Design review of the part built by this model. Coordinates are the model's own, in mm. A direction names the side the tool comes from. Coordinates: 2 decimals unless noted, no trailing zeros. Write each loop counter-clockwise with the first axis right and the second up, starting at its lowest first coordinate (ties: lowest second). Pieces come first, ordered by that corner, then holes. Notation, with made-up numbers: (-17, 84.25) -> (33, 84.25) arc R15 ccw to (33, 104.25) -> close; hole circle Ø4 at (76.25, 47.5). An arc over 180 degrees is marked (long way). Return JSON: item names as keys, results as strings. Group by question number.
from build123d import *

# Parameters (mm, degrees)
F0_R     = 3
F0_R_2   = 4.5
F1_DEPTH = 25


with BuildPart() as f1:
    # F0 (on Front) → F1 (new body)
    with BuildSketch(Plane.XZ):
        with BuildLine():
            ThreePointArc((10.9026810919, 60.0256923786), (-22.2558754476, 56.4666978044), (-51.1818335692, 39.870154161))
            ThreePointArc((-51.1818335692, 39.870154161), (-67.2310606154, 11.5408714989), (-71.6096891644, -20.7229403799))
            ThreePointArc((-71.6096891644, -20.7229403799), (-68.3273517642, -26.7421593589), (-61.4792606521, -27.0713766838))
            ThreePointArc((-61.4792606521, -27.0713766838), (-23.2487235956, -19.9089821225), (14.7948054645, -28.00612706))
            ThreePointArc((14.7948054645, -28.00612706), (34.09763812, -38.0650715452), (52.3656483576, -49.8998302939))
            ThreePointArc((52.3656483576, -49.8998302939), (55.6232730928, -50.3420263302), (57.6954634801, -47.7898344783))
            ThreePointArc((57.6954634801, -47.7898344783), (67.4841016349, -13.4719946795), (63.4264131289, 21.9831421749))
            ThreePointArc((63.4264131289, 21.9831421749), (41.7291215347, 47.3065311635), (10.9026810919, 60.0256923786))
        make_face()
        with Locations((-64.4427245231, -20.592329134)):
            Circle(F0_R, mode=Mode.SUBTRACT)
        with Locations((18.0438014374, -21.0330026143)):
            Circle(F0_R, mode=Mode.SUBTRACT)
        with Locations((-45.0222906279, 34.0597224955)):
            Circle(F0_R_2, mode=Mode.SUBTRACT)
        with BuildLine():
            add(Edge.make_bspline(
                [(-65.9818429495, -13.7766383887), (-64.3561406503, -13.9889919324), (-61.002475647, -14.4129805983), (-58.786662695, -17.3941098492), (-57.6425891256, -18.9315586575)],
                knots=[0, 0, 0, 0, 0.4837523045, 1, 1, 1, 1], degree=3))
            ThreePointArc((-65.9818429495, -13.7766383887), (-63.1199927656, 5.6889897511), (-55.6653674819, 23.8969393125))
            add(Edge.make_bspline(
                [(-55.6653674819, 23.8969393125), (-54.1157834703, 24.558722907), (-50.9743628562, 25.897077509), (-44.9169668051, 25.5411930836), (-44.499564984, 25.5987820264), (-44.4126954758, 25.6059592173)],
                knots=[0, 0, 0, 0, 0.4368464907, 0.8829086428, 1, 1, 1, 1], degree=3))
            ThreePointArc((-44.4126954758, 25.6059592173), (-38.3027773263, 28.8742935487), (-36.6900921562, 35.6131625664))
            add(Edge.make_bspline(
                [(-34.08346527, 45.6139450583), (-35.2318735073, 44.1052978146), (-37.495431158, 41.0832942182), (-36.9568434928, 37.4300314786), (-36.6900921562, 35.6131625664)],
                knots=[0, 0, 0, 0, 0.5034654691, 1, 1, 1, 1], degree=3))
            ThreePointArc((-34.08346527, 45.6139450583), (-21.4497726915, 51.0485334301), (-8.0636271487, 54.2038537692))
            add(Edge.make_bspline(
                [(-8.0636271487, 54.2038537692), (-5.1314488098, 53.9873966847), (0.3914162184, 53.5818086349), (3.3084081042, 49.9752607352), (4.6788664975, 48.2869338255)],
                knots=[0, 0, 0, 0, 0.5311112281, 1, 1, 1, 1], degree=3))
            ThreePointArc((4.6788664975, 48.2869338255), (8.9267083452, 46.2578656633), (13.5002491076, 47.3732144268))
            add(Edge.make_bspline(
                [(27.5275195375, 49.6756181297), (24.3589504651, 50.2644097694), (18.5753078163, 51.2779486411), (15.0780756623, 48.5877160028), (13.5002491076, 47.3732144268)],
                knots=[0, 0, 0, 0, 0.5497885765, 1, 1, 1, 1], degree=3))
            ThreePointArc((27.5275195375, 49.6756181297), (40.3031395338, 42.4916724249), (50.800144894, 32.2623801401))
            add(Edge.make_bspline(
                [(50.800144894, 32.2623801401), (51.3048604695, 30.5691603197), (52.2209505288, 27.262036777), (51.106083954, 24.3879103118), (50.5611791748, 22.9987592368)],
                knots=[0, 0, 0, 0, 0.5176067222, 1, 1, 1, 1], degree=3))
            ThreePointArc((50.5611791748, 22.9987592368), (50.2536306678, 17.192161847), (54.4628675293, 13.1804933194))
            add(Edge.make_bspline(
                [(61.7354629672, 6.576572241), (60.8612124825, 8.1098386582), (59.0540175823, 11.1146660647), (55.9863654121, 12.4994575374), (54.4628675293, 13.1804933194)],
                knots=[0, 0, 0, 0, 0.5060903587, 1, 1, 1, 1], degree=3))
            ThreePointArc((61.7354629672, 6.576572241), (61.8532031721, -17.8580596689), (54.0168535043, -41.0023186376))
            ThreePointArc((54.0168535043, -41.0023186376), (52.1556490377, -42.5112346478), (49.8949177563, -41.7175069451))
            ThreePointArc((49.8949177563, -41.7175069451), (40.3376909972, -35.0336152353), (30.4260621775, -28.8875103016))
            add(Edge.make_bspline(
                [(30.4260621775, -28.8875103016), (28.8541001513, -27.5081560411), (25.7225858464, -24.9527524994), (25.163523259, -21.2699310006), (24.8738721868, -19.4999880815)],
                knots=[0, 0, 0, 0, 0.5153021573, 1, 1, 1, 1], degree=3))
            ThreePointArc((24.8738721868, -19.4999880815), (20.7454507325, -14.5683653438), (14.3355783244, -15.0959089361))
            add(Edge.make_bspline(
                [(2.7973287746, -17.7149148802), (5.5242069664, -17.7559248974), (10.3675947849, -17.828765488), (13.1289117857, -15.9269725037), (14.3355783244, -15.0959089361)],
                knots=[0, 0, 0, 0, 0.5630104988, 1, 1, 1, 1], degree=3))
            ThreePointArc((2.7973287746, -17.7149148802), (-27.4894908213, -15.0017617251), (-57.6425891256, -18.9315586575))
        make_face(mode=Mode.SUBTRACT)
        with Locations((56.7802422866, 19.7857771311)):
            Circle(F0_R, mode=Mode.SUBTRACT)
        with Locations((9.6443155061, 53.228250787)):
            Circle(F0_R, mode=Mode.SUBTRACT)
    extrude(amount=F1_DEPTH)


solid = f1.part
Q1. We need section C-C on x = -42.5. Write out the cut boundary in (y, z), plus the area to 3 significant figures.
Q2. We need section A-A on z = -38. Write out the cut boundary in (x, y), plus the area to 3 significant figures.
Q3. Wall thickness on L1, parallel to Z at x = -42.5, y = -8.75; L2, parallel to Z at x = -46, y = -10.5; L3, parallel to Z at x = -15, y = -14.5: over which ranges is each line inside the solid? List them lowest first.
Q4. For faces 5 (the flat face through (-2, 0, -19)), 6 (the cylindrical face through (-27.063, -12.325, -14.994)), list the 3-axis set-ups (+Z, -Z, +X, -X, +Y, -Y) from which the entire face can be reached by the end or side of a thin tool; tool diameter is ignored.
Q5. The part is to be moulded in two halves that separate along X. For faces 1 (the flat face through (-2, -25, -19)), 2 (the cylindrical face through (67.44, -12.32, -13.97)), 3 (the cylindrical face through (-38.36, -12.32, 28.8)), 4 (the cylindrical face through (61.907, -12.325, -17.519)), say which applies: +X half, -X half, draft (parallel to the pull), parting line (faces both ways), or undercut.
Q6. We need section B-B on x = -28.5. Write out the cut boundary in (y, z).
Q7. We need section D-D on y = -6. State how many separate pieces and enclosed holes the cut face has, plus the area to 3 significant figures.
Q8. For P1, Ø3, axis at x = -16, y = -5, coming from the +Z side; P2, Ø2, axis at y = -6.5, z = -3.5, coming from the -X side; P3, Ø6, axis at x = 17.5, y = -22, coming from the -Z side; P4, Ø5, axis at x = -37.5, z = -20, coming from the +Y side, all flat-tipped, find the tip position at first contact; note any pin that passes through.
Findings below:
{
 "1": {"outline": "(-25, -21.56) -> (0, -21.56) -> (0, -16.12) -> (-25, -16.12) -> close; (-25, 25.96) -> (0, 25.96) -> (0, 30.33) -> (-25, 30.33) -> close; (-25, 37.79) -> (0, 37.79) -> (0, 46.61) -> (-25, 46.61) -> close", "area": "466 mm^2"},
 "2": {"outline": "(33.99, -25) -> (44.72, -25) -> (44.72, 0) -> (33.99, 0) -> close; (55.54, -25) -> (62.01, -25) -> (62.01, 0) -> (55.54, 0) -> close", "area": "430 mm^2"},
 "3": {"L1": "z = -21.56 to -16.12, 25.96 to 30.33, 37.79 to 46.61", "L2": "z = -22.27 to -16.62, 25.61 to 29.67, 38.45 to 44.12", "L3": "z = -20.35 to -15.31, 52.88 to 58.46"},
 "4": {"face 5": "+Z, -Z, +X, -X, +Y", "face 6": "+Y, -Y"},
 "5": {"face 1": "draft", "face 2": "+X half", "face 3": "undercut", "face 4": "undercut"},
 "6": {"outline": "(-25, -19.98) -> (0, -19.98) -> (0, -15.03) -> (-25, -15.03) -> close; (-25, 48.34) -> (0, 48.34) -> (0, 54.15) -> (-25, 54.15) -> close"},
 "7": {"separate pieces": "1", "enclosed holes": "6", "area": "2,590 mm^2"},
 "8": {"P1": "stops at z = 58.57", "P2": "stops at x = -70.98", "P3": "stops at z = -30.74", "P4": "stops at y = 0"}
}
